```python
from build123d import *

# Parameters (mm, degrees)
SKETCH_1_R                      = 2.75
EXTRUDE_1_DEPTH                 = 7
CUT_EXTRUDE_1_DEPTH             = 6
EXTRUDE_2_DEPTH                 = 3.5
EXTRUDE_START                   = -4
SKETCH_5_R                      = 5
SKETCH_5_R_2                    = 2.75
EXTRUDE_3_DEPTH                 = 4
SWEEP_1_PROFILE_R               = 1.25
CUT_EXTRUDE_2_REACH             = 12.308
SKETCH_13_R                     = 0.9
CUT_EXTRUDE_2_DIRECTION_2_REACH = 12.308


with BuildPart() as part:
    # 草图1 → 凸台-拉伸1 (new body)
    with BuildSketch(Plane(origin=(0, 0, 0), x_dir=(1, 0, 0), z_dir=(0, 1, 0))):
        with Locations(Location((0, 0, 0), (0, 0, 270))):
            Circle(SKETCH_1_R)
    extrude(amount=EXTRUDE_1_DEPTH)

    # 草图2 → 切除-拉伸1 (cut)
    with BuildSketch(Plane(origin=(0, 7, 0), x_dir=(1, 0, 0), z_dir=(0, 1, 0))):
        with BuildLine():
            Line((1.843908891, 1.2), (-1.843908891, 1.2))
            ThreePointArc((-1.843908891, 1.2), (-2.2, 0), (-1.843908891, -1.2))
            Line((-1.843908891, -1.2), (1.843908891, -1.2))
            ThreePointArc((1.843908891, -1.2), (2.109099282, -0.625859584), (2.2, 0))
            ThreePointArc((2.2, 0), (2.109099282, 0.625859584), (1.843908891, 1.2))
        make_face()
    extrude(amount=-CUT_EXTRUDE_1_DEPTH, mode=Mode.SUBTRACT)

    # 草图4 → 凸台-拉伸2 (add)
    with BuildSketch(Plane(origin=(0, 7, 0), x_dir=(1, 0, 0), z_dir=(0, 1, 0))):
        with BuildLine():
            ThreePointArc((1.6, 1.2), (0, 2), (-1.6, 1.2))
            Line((-1.6, 1.2), (1.6, 1.2))
        make_face()
        with BuildLine():
            ThreePointArc((-1.6, -1.2), (0, -2), (1.6, -1.2))
            Line((1.6, -1.2), (-1.6, -1.2))
        make_face()
    extrude(amount=EXTRUDE_2_DEPTH)

    # 草图5 → 凸台-拉伸3 (add)
    with BuildSketch(Plane(origin=(0, 7, 0), x_dir=(1, 0, 0), z_dir=(0, 1, 0)).offset(EXTRUDE_START)):
        with Locations(Location((0, 0, 0), (0, 0, 270))):
            Circle(SKETCH_5_R)
        with Locations(Location((0, 0, 0), (0, 0, 270))):
            Circle(SKETCH_5_R_2, mode=Mode.SUBTRACT)
    extrude(amount=EXTRUDE_3_DEPTH)

    # 切除-扫描1: sweep along a path in 草图6
    with BuildLine(Plane(origin=(0, 5, 0), x_dir=(-1, 0, 0), z_dir=(0, -1, 0))) as sweep_1_path:
        CenterArc((0, 0), 4.3, 0, 360)
    # 切除-扫描1 profile (on start of the path) → 切除-扫描1 (sweep, cut)
    with BuildSketch(Plane(origin=(-4.3, 5, 0), x_dir=(-1, 0, 0), z_dir=(0, 0, -1))):
        Circle(SWEEP_1_PROFILE_R)
    sweep(path=sweep_1_path.line, mode=Mode.SUBTRACT)

    # 草图13 → 切除-拉伸2 (cut, up to next)
    with BuildSketch(Plane.XZ.offset(-3), mode=Mode.PRIVATE) as cut_extrude_2_sk1:
        with Locations(Location((0, 3, 0), (0, 0, 90))):
            Circle(SKETCH_13_R)
    cut_extrude_2_tool1 = extrude(cut_extrude_2_sk1.sketch, amount=-CUT_EXTRUDE_2_REACH, mode=Mode.PRIVATE) & part.part
    # 草图13 → 切除-拉伸2 (cut, up to next)
    with BuildSketch(Plane.XZ.offset(-3), mode=Mode.PRIVATE) as cut_extrude_2_sk2:
        with Locations(Location((0, -3, 0), (0, 0, 90))):
            Circle(SKETCH_13_R)
    cut_extrude_2_tool2 = extrude(cut_extrude_2_sk2.sketch, amount=-CUT_EXTRUDE_2_REACH, mode=Mode.PRIVATE) & part.part
    add(cut_extrude_2_tool1.solids().sort_by_distance((0, 3, 3))[0], mode=Mode.SUBTRACT)
    add(cut_extrude_2_tool2.solids().sort_by_distance((0, 3, -3))[0], mode=Mode.SUBTRACT)

    # 草图13 → 切除-拉伸2 direction 2 (cut, up to next)
    with BuildSketch(Plane.XZ.offset(-3), mode=Mode.PRIVATE) as cut_extrude_2_direction_2_sk1:
        with Locations(Location((0, 3, 0), (0, 0, 90))):
            Circle(SKETCH_13_R)
    cut_extrude_2_direction_2_tool1 = extrude(cut_extrude_2_direction_2_sk1.sketch, amount=CUT_EXTRUDE_2_DIRECTION_2_REACH, mode=Mode.PRIVATE) & part.part
    # 草图13 → 切除-拉伸2 direction 2 (cut, up to next)
    with BuildSketch(Plane.XZ.offset(-3), mode=Mode.PRIVATE) as cut_extrude_2_direction_2_sk2:
        with Locations(Location((0, -3, 0), (0, 0, 90))):
            Circle(SKETCH_13_R)
    cut_extrude_2_direction_2_tool2 = extrude(cut_extrude_2_direction_2_sk2.sketch, amount=CUT_EXTRUDE_2_DIRECTION_2_REACH, mode=Mode.PRIVATE) & part.part
    add(cut_extrude_2_direction_2_tool1.solids().sort_by_distance((0, 3, 3))[0], mode=Mode.SUBTRACT)
    add(cut_extrude_2_direction_2_tool2.solids().sort_by_distance((0, 3, -3))[0], mode=Mode.SUBTRACT)


solid = part.part
```
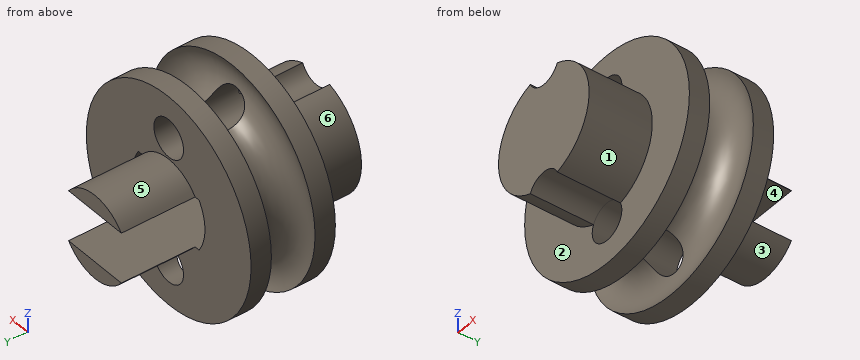
Can you work these out from the model? Positions are in its coordinate system, mm. Face numbers are marked on the shaded views. A direction names the side the tool comes from. Round coordinates to 2 decimals unless told otherwise and drop trailing zeros. Loops run counter-clockwise (first coordinate to the right, second up) from the corner with the lowest first, then second, coordinate; pieces in that order, holes last. Notation, with made-up numbers: M -7,-12 L 31,-12 A24 cw 31,3 Z; hole C 78,28.5 d7. An arc over 180 degrees is marked long. Write item = value, one per line. Start each with the question number.
(1) Suppose I cut it at C-C on y = 8.75. Write out the boundary of the cut face in (x, z), plus the area to 3 significant figures.
(2) Suppose I cut it at B-B on x = 0. Write out the boundary of the cut face in (y, z).
(3) I need wall thicknesses on line 1 along Z through (x, y) = (0.75, 3.25); line 2 along Z through (x, y) = (0, 2.75); line 3 along X through (y, z) = (4.5, 1.75). Which ranges of each line are inside material? Lowest first, please.
(4) Suppose I cut it at D-D on z = 3. Give the number of separate pieces and of enclosed holes in the cut face, plus the area to 3 significant figures.
(5) If we mould it in two halves opening along X, with no side actions, what happens to the marked faces 4, 5 and 6? For each: released by +X, released by -X, zero draft, split by the parting line, or undercut.
(6) Which directions (+Z, -Z, +X, -X, +Y, -Y) give clear straight access to the entire face, cutting with the end or side of a thin tool? Please do the marked faces 1, 2 and 3.
(7) Suppose I cut it at A-A on y = 6.5. Write out the boundary of the cut face in (x, z).
(8) I'm going to push flat-ended pins straight in: P1, Ø1.5, axis at x = -3.5, y = 9.5, coming from the -Z side; P2, Ø1, axis at x = -2, y = 4.5, coming from the +Z side. Where does each tip first touch, or does it pass through?
Answer block:
q1.outline = M -1.6,-1.2 A2 ccw 1.6,-1.2 Z; M -1.6,1.2 L 1.6,1.2 A2 ccw Z
q1.area = 3.58 mm²
q2.outline = M 0,-2.1 L 7,-2.1 L 7,-2 L 10.5,-2 L 10.5,-1.2 L 1,-1.2 L 1,1.2 L 10.5,1.2 L 10.5,2 L 7,2 L 7,2.1 L 0,2.1 Z; M 3,-5 L 3.96,-5 A1.25 cw 3.82,-3.9 L 3,-3.9 Z; M 3,3.9 L 3.82,3.9 A1.25 cw 3.96,5 L 3,5 Z; M 6.04,-5 L 7,-5 L 7,-3.9 L 6.18,-3.9 A1.25 cw Z; M 6.04,5 A1.25 cw 6.18,3.9 L 7,3.9 L 7,5 Z
q3.line_1 = -4.94 to -3.5, -2.5 to -1.2, 1.2 to 2.5, 3.5 to 4.94
q3.line_2 = -2.1 to -1.2, 1.2 to 2.1
q3.line_3 = -2.62 to 2.62
q4.separate_pieces = 4
q4.enclosed_holes = 0
q4.area = 11.9 mm²
q5.face_4 = undercut
q5.face_5 = split by the parting line
q5.face_6 = released by -X
q6.face_1 = +X, -Y
q6.face_2 = -Y
q6.face_3 = -Z, +Y
q7.outline = C 0,0 d10; hole M -1.84,-1.2 L 1.84,-1.2 A2.2 ccw 1.84,1.2 L -1.84,1.2 A2.2 ccw Z; hole C 0,-3 d1.8; hole C 0,3 d1.8
q8.P1 = through
q8.P2 = 3
